Geometry: final body of the model. Coordinates: model frame, mm. A direction names the side the tool comes from. Give positions to 0.01 mm unless a question says otherwise; leave off trailing zeros. Order: outer loops, then holes, each group sorted by start corner. A loop starts at its lowest first (then second) coordinate and runs counter-clockwise, first axis right, second up. Notation, with made-up numbers: (27, 49.25) - (51, 49.25) arc R23 cw to (51, 78.25) - close; hole circle Ø7 at (-10, 20). An arc over 180 degrees is marked (long way). Write item = value, one per line. Start each with the question number.
from build123d import *

# Parameters (mm, degrees)
BOSS_EXTRUDE1_DEPTH = 15
SKETCH4_R           = 5
CUT_EXTRUDE1_DEPTH  = 267.176633084
SKETCH5_R           = 7.5
CUT_EXTRUDE2_DEPTH  = 267.176633084


with BuildPart() as part:
    # Sketch1 → Boss-Extrude1 (new body)
    with BuildSketch(Plane(origin=(0, 0, 0), x_dir=(1, 0, 0), z_dir=(0, 1, 0))):
        Polygon((-200, -175), (200, -175), (200, -109.36837475), (192.446978441, -109.36837475), (192.446978441, -34.36837475), (200, -34.36837475), (200, 175), (-200, 175), (-200, -34.36837475), (-192.446978441, -34.36837475), (-192.446978441, -109.36837475), (-200, -109.36837475), align=None)
    extrude(amount=BOSS_EXTRUDE1_DEPTH)

    # Sketch4 → Cut-Extrude1 (cut, through all)
    with BuildSketch(Plane(origin=(0, 15, 0), x_dir=(1, 0, 0), z_dir=(0, 1, 0))):
        with Locations(Location((-170, 148.75, 0), (0, 0, 270))):
            Circle(SKETCH4_R)
        with Locations(Location((170, 148.75, 0), (0, 0, 90))):
            Circle(SKETCH4_R)
        with Locations(Location((170, -148.75, 0), (0, 0, 270))):
            Circle(SKETCH4_R)
        with Locations(Location((-170, -148.75, 0), (0, 0, 90))):
            Circle(SKETCH4_R)
        Polygon((-170, 175), (-200, 145), (-200, 175), align=None)
        Polygon((-200, -145), (-200, -175), (-170, -175), align=None)
        Polygon((170, -175), (200, -145), (200, -175), align=None)
        Polygon((200, 145), (200, 175), (170, 175), align=None)
    extrude(amount=-CUT_EXTRUDE1_DEPTH, mode=Mode.SUBTRACT)

    # Sketch5 → Cut-Extrude2 (cut, through all)
    with BuildSketch(Plane.XZ):
        with Locations(Location((0, -135, 0), (0, 0, 270))):
            Circle(SKETCH5_R)
    extrude(amount=-CUT_EXTRUDE2_DEPTH, mode=Mode.SUBTRACT)


solid = part.part
Q1. Material intervals for line 1 along X through (y, z) = (8.25, 149); line 2 along X through (y, z) = (9.25, -148.75); line 3 along Z through (x, y) = (2.5, 10.5), sorted ascending. Write a range as from..to.
Q2. Contact query for flat-ended pins moving along their axis: pin 1 (4.5 mm diameter, centred on y = 6, z = 80, fed in from +X); pin 2 (4 mm diameter, centred on x = -195.5, y = 11, fed in from -Z); pin 3 (4 mm diameter, centred on x = 197.5, y = 5.5, fed in from +Z). Output: stop coordinate, or through.
Q3. Pull-direction query (X, two-part tool) for faces 1 (the flat face through (-3, 0, -2)), 2 (the flat face through (-200, 7, -57)), 3 (the cylindrical face through (165.043, 7.605, -148.099)); classes: +X half, -X half, draft (parallel to the pull), parting line (faces both ways), or undercut.
Q4. Set-up query: faces 4 (the flat face through (-192.447, 7, 71)), 5 (the flat face through (185, 8, 160)), 6 (the flat face through (192.447, 7, 72)). Return all of +Z, -Z, +X, -X, +Y, -Y with unobstructed straight access to the full face (end or side cutting, diameter ignored); none if empty.
Q5. Section A-A, the plane y = 8. Return the cut outline in (x, z), then the cut area to 3 significant figures.
Q6. Section C-C, the plane z = -135. Return the cut outline in (x, y).
Q7. Section D-D, the plane z = 87. Return the cut outline in (x, y).
Q8. Section B-B, the plane x = 0. Return the cut outline in (y, z).
The answers:
q1.line_1 = -196..-174.99, -165.01..165.01, 174.99..196
q1.line_2 = -196.25..-175, -165..165, 175..196.25
q1.line_3 = -175..-142.07, -127.93..175
q2.pin_1 = 192.45
q2.pin_2 = -151.5
q2.pin_3 = 149.5
q3.face_1 = draft
q3.face_2 = -X half
q3.face_3 = undercut
q4.face_4 = -X, +Y, -Y
q4.face_5 = +Z, +X, +Y, -Y
q4.face_6 = +X, +Y, -Y
q5.outline = (-200, -145) - (-170, -175) - (170, -175) - (200, -145) - (200, 34.37) - (192.45, 34.37) - (192.45, 109.37) - (200, 109.37) - (200, 145) - (170, 175) - (-170, 175) - (-200, 145) - (-200, 109.37) - (-192.45, 109.37) - (-192.45, 34.37) - (-200, 34.37) - close; hole circle Ø10 at (-170, -148.75); hole circle Ø10 at (-170, 148.75); hole circle Ø15 at (0, -135); hole circle Ø10 at (170, -148.75); hole circle Ø10 at (170, 148.75)
q5.area = 137,000 mm²
q6.outline = (-200, 0) - (-7.5, 0) - (-7.5, 15) - (-200, 15) - close; (7.5, 0) - (200, 0) - (200, 15) - (7.5, 15) - close
q7.outline = (-192.45, 0) - (192.45, 0) - (192.45, 15) - (-192.45, 15) - close
q8.outline = (0, -175) - (15, -175) - (15, -142.5) - (0, -142.5) - close; (0, -127.5) - (15, -127.5) - (15, 175) - (0, 175) - close
